from build123d import *

# Parameters (mm, degrees)
BOSS_EXTRUDE1_DEPTH = 6
CUT_EXTRUDE1_REACH  = 30.66
SKETCH3_R           = 1.5
BOSS_EXTRUDE2_DEPTH = 5.75
CUT_EXTRUDE2_START  = 6.25
CUT_EXTRUDE2_DEPTH  = 6.25
CHAMFER1_SIZE       = 1
FILLET1_R           = 10
SKETCH7_W           = 2
SKETCH7_H           = 12
BOSS_EXTRUDE3_DEPTH = 6
SKETCH8_W           = 6.2
SKETCH8_H           = 6.2
CUT_EXTRUDE3_DEPTH  = 2


with BuildPart() as part:
    # Sketch2 → Boss-Extrude1 (new, symmetric)
    with BuildSketch(Plane(origin=(0, 0, 0), x_dir=(1, 0, 0), z_dir=(0, 1, 0))):
        with BuildLine():
            Line((6, 6.75), (-14.2, 6.75))
            Line((-14.2, 6.75), (-14.2, 0))
            Line((-14.2, 0), (-16.2, 0))
            ThreePointArc((-16.2, 0), (-20.7, 4.5), (-25.2, 0))
            Line((-25.2, 0), (-27.2, 0))
            ThreePointArc((-27.2, 0), (-26.012050082, 3.745947667), (-22.882423407, 6.122665112))
            ThreePointArc((-22.882423407, 6.122665112), (-16.536777753, 7.78906592), (-10, 8.35))
            Line((-10, 8.35), (6, 8.35))
            Line((6, 8.35), (6, 6.75))
        make_face()
    extrude(amount=BOSS_EXTRUDE1_DEPTH, both=True)

    # Sketch3 → Cut-Extrude1 (cut, up to next)
    with BuildSketch(Plane.XY.offset(-6.75), mode=Mode.PRIVATE) as cut_extrude1_sk1:
        Circle(SKETCH3_R)
    cut_extrude1_tool1 = extrude(cut_extrude1_sk1.sketch, amount=-CUT_EXTRUDE1_REACH, mode=Mode.PRIVATE) & part.part
    add(cut_extrude1_tool1.solids().sort_by_distance((0, 0, -6.75))[0], mode=Mode.SUBTRACT)

    # Sketch5 → Boss-Extrude2 (add)
    with BuildSketch(Plane(origin=(0, -0.25, 0), x_dir=(1, 0, 0), z_dir=(0, 1, 0))):
        with BuildLine():
            Line((-24.928616794, -1.539090645), (-26.808002035, -2.223130932))
            ThreePointArc((-26.808002035, -2.223130932), (-21.828713155, 6.401250395), (-14.2, 0))
            Line((-14.2, 0), (-14.2, -2.365806523))
            Line((-14.2, -2.365806523), (-16.471383206, -1.539090645))
            ThreePointArc((-16.471383206, -1.539090645), (-20.7, 4.5), (-24.928616794, -1.539090645))
        make_face()
    extrude(amount=-BOSS_EXTRUDE2_DEPTH)

    # Sketch6 → Cut-Extrude2 (cut)
    with BuildSketch(Plane(origin=(0, -0.25, 0), x_dir=(1, 0, 0), z_dir=(0, 1, 0)).offset(CUT_EXTRUDE2_START)):
        with BuildLine():
            Line((-24.901111919, 1.612655773), (-26.768272772, 2.329391672))
            ThreePointArc((-26.768272772, 2.329391672), (-21.884530916, -6.391156899), (-14.2, 0))
            Line((-14.2, 0), (-14.2, 2.495116228))
            Line((-14.2, 2.495116228), (-16.498888081, 1.612655773))
            ThreePointArc((-16.498888081, 1.612655773), (-20.7, -4.5), (-24.901111919, 1.612655773))
        make_face()
    extrude(amount=-CUT_EXTRUDE2_DEPTH, mode=Mode.SUBTRACT)

    # Chamfer1
    chamfer1_edges = [part.edges().sort_by_distance(p)[0] for p in [
        (-20.7, -6, -4.5),
        (-20.7, 6, -4.5),
    ]]
    chamfer(chamfer1_edges, length=CHAMFER1_SIZE)

    # Fillet1
    # the kernel refuses this fillet: 10 mm, written as the material it takes off along each edge
    with BuildSketch(Plane(origin=(-20.7, -5, 0), x_dir=(0.003141587485880374, 0, 0.9999950652018581), z_dir=(-0.9999950652018581, 0, 0.003141587485880374))) as fillet1_piece_1:
        with BuildLine():
            CenterArc((14.5, 3.358898944), FILLET1_R, 180, 25.841932763)
            Line((5.5, -1), (5.32, -1.087177979))
            ThreePointArc((5.32, -1.087177979), (4.858578644, -0.641421356), (4.358578644, -0.141421356))
            Line((4.358578644, -0.141421356), (4.3, 0))
            Line((4.3, 0), (4.3, 3.358898944))
            Line((4.3, 3.358898944), (4.5, 3.358898944))
        make_face()
    revolve(axis=Axis((-20.7, -5, 0), (0, 1, 0)), revolution_arc=359.64, mode=Mode.SUBTRACT)
    with BuildSketch(Plane(origin=(-20.7, 5, 0), x_dir=(0.06944148542988178, 0, 0.9975860264164146), z_dir=(-0.9975860264164146, 0, 0.06944148542988178))) as fillet1_piece_2:
        with BuildLine():
            CenterArc((14.5, -3.358898944), FILLET1_R, 154.158067237, 25.841932763)
            Line((5.5, 1), (5.32, 1.087177979))
            ThreePointArc((5.32, 1.087177979), (4.858578644, 0.641421356), (4.358578644, 0.141421356))
            Line((4.358578644, 0.141421356), (4.3, 0))
            Line((4.3, 0), (4.3, -3.358898944))
            Line((4.3, -3.358898944), (4.5, -3.358898944))
        make_face()
    revolve(axis=Axis((-20.7, 5, 0), (0, 1, 0)), revolution_arc=352.036182743, mode=Mode.SUBTRACT)

    # Sketch7 → Boss-Extrude3 (add, symmetric)
    with BuildSketch(Plane(origin=(0, 0, 0), x_dir=(0, 0, -1), z_dir=(1, 0, 0))):
        with Locations((9.35, 0)):
            Rectangle(SKETCH7_W, SKETCH7_H)
    extrude(amount=BOSS_EXTRUDE3_DEPTH, both=True)

    # Sketch8 → Cut-Extrude3 (cut)
    with BuildSketch(Plane(origin=(0, 0, -10.35), x_dir=(-1, 0, 0), z_dir=(0, 0, -1))):
        Rectangle(SKETCH8_W, SKETCH8_H)
    extrude(amount=-CUT_EXTRUDE3_DEPTH, mode=Mode.SUBTRACT)


solid = part.part
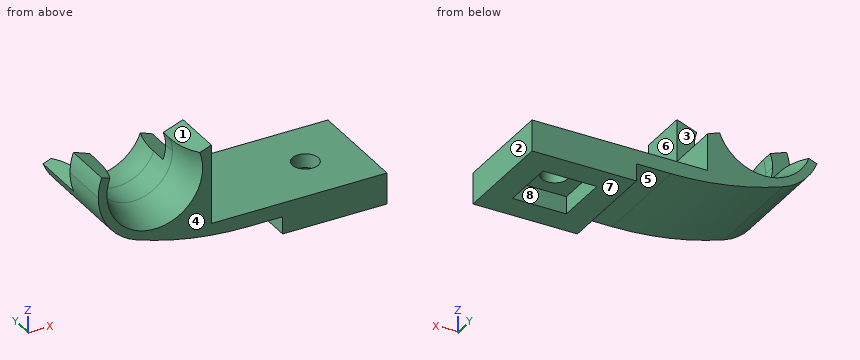
Model file for the job. Use its own axes, mm. Face numbers are marked on the shaded views. A direction names the side the tool comes from. Give positions to 0.01 mm unless a question says otherwise; leave off trailing zeros. Write each loop counter-clockwise with the first axis right and the second up, starting at its lowest first coordinate (ties: lowest second). Pieces come first, ordered by that corner, then holes. Notation, with made-up numbers: (37, 81) - (50, 81) arc R22 cw to (50, 94) - close; hole circle Ø5 at (39, -23.75). An arc over 180 degrees is marked (long way). Answer as CSV lines item,"result".
1. Drill centre lines: L1, parallel to Y at x = 0, z = -7.55; L2, parallel to Z at x = 2, y = 0.75; L3, parallel to Z at x = 1.5, y = -5.25. Where is each one in solid material? Low to high. Write a range as [from, to].
Responses:
L1,"y = [-6, -1.5], [1.5, 6]"
L2,"z = [-8.35, -6.75]"
L3,"z = [-10.35, -6.75]"
2. Band-saw the part on A-A (x = 0). Write the cut outline in (y, z).
Responses:
outline,"(-6, -10.35) - (-3.1, -10.35) - (-3.1, -8.35) - (-1.5, -8.35) - (-1.5, -6.75) - (-6, -6.75) - close; (1.5, -8.35) - (3.1, -8.35) - (3.1, -10.35) - (6, -10.35) - (6, -6.75) - (1.5, -6.75) - close"
3. Two-plate mould, pull along X, no slides. Class the marked faces 1, 2 and 3: +X half, -X half, draft (parallel to the pull), parting line (faces both ways), or undercut.
Responses:
face 1,"undercut"
face 2,"+X half"
face 3,"draft"
4. 3-axis set-ups, long thin cutter, end or side, ignore diameter. For the marked faces 4, 5, 6, 7 and 8: which of +Z, -Z, +X, -X, +Y, -Y reach the whole face in a straight line?
Responses:
face 4,"+Z, -Z, +X, -X, -Y"
face 5,"-Z, -X, +Y, -Y"
face 6,"+Z, +X, +Y, -Y"
face 7,"-Z, +X, -X, +Y, -Y"
face 8,"-Z"
5. Band-saw the part on D-D (y = -4.5). Write the cut outline in (x, z), and give its area (3 significant figures).
Responses:
outline,"(-26.81, 2.22) arc R6.5 ccw to (-22.88, -6.12) arc R38.37 ccw to (-10, -8.35) - (-6, -8.35) - (-6, -10.35) - (6, -10.35) - (6, -6.75) - (-14.2, -6.75) - (-14.2, 2.37) - (-16.08, 1.68) arc R4.92 cw (long way) to (-25.32, 1.68) - close"
area,"107 mm2"
6. Band-saw the part on C-C (z = -7.5). Write the cut outline in (x, y).
Responses:
outline,"(-18.03, -6) - (6, -6) - (6, 6) - (-18.03, 6) - close; hole circle Ø3 at (0, 0)"
7. Band-saw the part on B-B (y = 0.75). Write the cut outline in (x, z).
Responses:
outline,"(-26.77, -2.33) arc R6.5 ccw to (-22.88, -6.12) arc R38.37 ccw to (-10, -8.35) - (-6, -8.35) - (-6, -10.35) - (-3.1, -10.35) - (-3.1, -8.35) - (-1.3, -8.35) - (-1.3, -6.75) - (-14.2, -6.75) - (-14.2, -2.5) - (-16.5, -1.61) arc R4.5 cw to (-24.9, -1.61) - close; (1.3, -8.35) - (3.1, -8.35) - (3.1, -10.35) - (6, -10.35) - (6, -6.75) - (1.3, -6.75) - close"
8. Pin check, flat tips, straight feed: pin 1 (1.5 mm diameter, centred on x = -23.5, z = -3.5, fed in from +Y); pin 2 (4.5 mm diameter, centred on y = -2.5, z = -3.5, fed in from +X); pin 3 (2 mm diameter, centred on y = 1, z = -9.5, fed in from -X). Stop position of each tip, or through.
Responses:
pin 1,"stops at y = 5.4"
pin 2,"stops at x = -14.2"
pin 3,"stops at x = -6"
